Can you work these out from the model? Positions are in its coordinate system, mm. Give positions to 0.01 mm unless a question says otherwise; leave off trailing zeros. Order: outer loops, then holes, each group sorted by start corner. A loop starts at its lowest first (then second) coordinate and runs counter-clockwise, first axis right, second up. Notation, with made-up numbers: (63, 6.5) - (111, 6.5) arc R16 ccw to (111, 24.5) - close; hole circle Ø1 at (51, -4). An arc over 180 degrees is marked (long way). Answer as a JSON object with one key per item and string values.
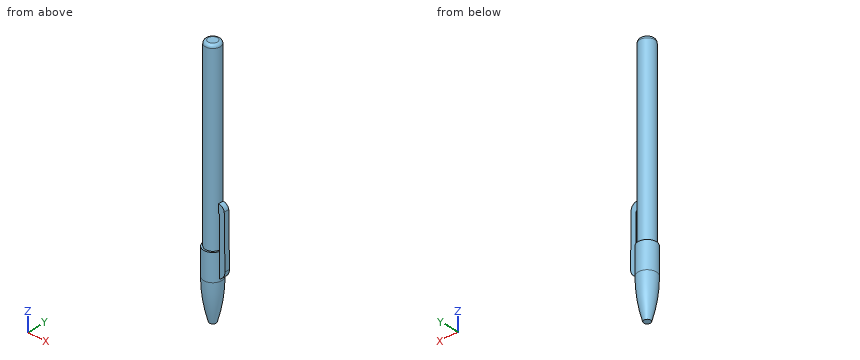
Solid Edge part; units mm, degrees
sketch "Sketch1" plane through (0, 0, 0) normal (0, -1, 0) x (1, 0, 0)
  line L0 (0, 149) -> (4.5, 149)
  line L1 (4.5, 149) -> (4.5, 40)
  line L2 (4.5, 40) -> (5.5, 40)
  line L3 (5.5, 40) -> (5.5, 24)
  arc A0 (5.5, 24) -> (2, 0) centre (-78.5357, 24) cw
  line L4 (2, 0) -> (0, 0)
  dimension "D1" = 4.5
  dimension "D2" = 5.5
  dimension "D3" = 2
revolve "RevolvedProtrusion1" add sketch "Sketch1" angle 360 about axis through (0, 0, 0) along (0, 0, 1)
sketch "Sketch2" plane through (0, 0, 0) normal (0, -1, 0) x (1, 0, 0)
  line L0 (5.5, 40) -> (5.5, 59.6951)
  line L1 (5.5, 59.6951) -> (4.8296, 60.1792)
  line L2 (4.8296, 60.1792) -> (4.8296, 65.0875)
  arc A0 (4.8296, 65.0875) -> (8.2936, 62.077) centre (4.8296, 61.5894) cw
  line L3 (8.2936, 62.077) -> (8.7357, 30.6437)
  arc A1 (8.7357, 30.6437) -> (5.5, 25.5622) centre (3.249, 30.5665) cw
  line L4 (3.5, 25.5622) -> (5.5, 25.5622)
  line L5 (3.5, 40) -> (3.5, 25.5622)
  line L6 (5.5, 40) -> (3.5, 40)
  dimension "D1" = 3.5
extrude "Protrusion1" add sketch "Sketch2" along normal mid plane 3
fillet "Round_1" radius 1.75 1 edges at (-4.5, 0, 149)
Q1. If we section it at A-A, the plane x = 7: Please give me the cut outline in (y, z).
Recorded:
{"outline": "(-1.5, 26.56) - (1.5, 26.56) - (1.5, 64.33) - (-1.5, 64.33) - close"}
Q2. I'm going to push flat-ended pins straight in: pin 1 Ø1 at (y, z) = (-3, 105.5) entering from +X; pin 2 Ø2 at (x, z) = (7, 44.5) entering from +Y; pin 3 Ø2 at (x, z) = (6, 44) entering from -Y. Where does each tip first touch, or does it pass through?
Recorded:
{"pin 1": "stops at x = 3.74", "pin 2": "stops at y = 1.5", "pin 3": "stops at y = -1.5"}
Q3. I need wall thicknesses on L1, parallel to Y at x = 0, z = 118.5; L2, parallel to X at y = 0.25, z = 32; L3, parallel to X at y = 1.25, z = 139.5. Which ranges of each line are inside material? Lowest first, please.
Recorded:
{"L1": "y = -4.5 to 4.5", "L2": "x = -5.49 to 8.72", "L3": "x = -4.32 to 4.32"}
